Verification items for the finished model (mm, model axes). Face numbers are marked on the shaded views. A direction names the side the tool comes from. Round coordinates to 2 decimals unless told otherwise and drop trailing zeros. Loops run counter-clockwise (first coordinate to the right, second up) from the corner with the lowest first, then second, coordinate; pieces in that order, holes last. Notation, with made-up numbers: (19.5, -19.75) - (26.5, -19.75) arc R30 ccw to (26.5, 12.25) - close; hole circle Ø7 at (82, -11). An arc over 180 degrees is marked (long way). Use a Markdown table: item, result. Add a question column.
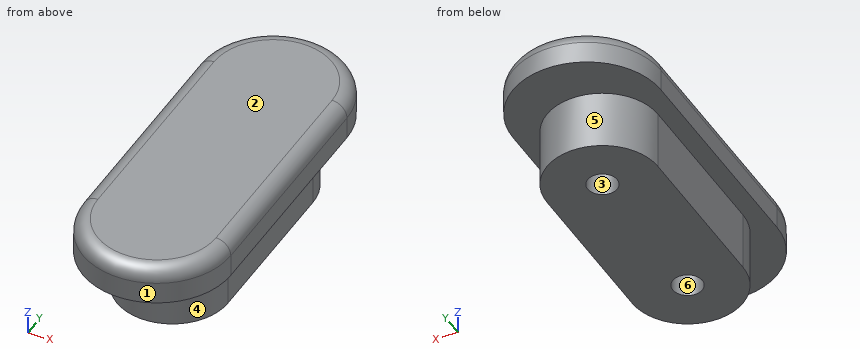
```python
from build123d import *

# Parameters (mm, degrees)
SKETCH_2_R      = 2
EXTRUDE_1_DEPTH = 8
EXTRUDE_2_DEPTH = 5
FILLET_1_R      = 2


with BuildPart() as part:
    # 草图2 → 凸台-拉伸1 (new body)
    with BuildSketch(Plane.XY):
        with BuildLine():
            Line((-7.5, -11), (-7.5, 11))
            ThreePointArc((-7.5, 11), (0, 18.5), (7.5, 11))
            Line((7.5, 11), (7.5, -11))
            ThreePointArc((7.5, -11), (0, -18.5), (-7.5, -11))
        make_face()
        with Locations((0, -11)):
            Circle(SKETCH_2_R, mode=Mode.SUBTRACT)
        with Locations((0, 11)):
            Circle(SKETCH_2_R, mode=Mode.SUBTRACT)
    extrude(amount=EXTRUDE_1_DEPTH)

    # 草图3 → 凸台-拉伸2 (add)
    with BuildSketch(Plane.XY.offset(8)):
        with BuildLine():
            Line((-10, -15), (-10, 15))
            ThreePointArc((-10, 15), (0, 25), (10, 15))
            Line((10, 15), (10, -15))
            ThreePointArc((10, -15), (0, -25), (-10, -15))
        make_face()
    extrude(amount=EXTRUDE_2_DEPTH)

    # 圆角1
    fillet_1_edges = [part.edges().sort_by_distance(p)[0] for p in [
        (0, -25, 13),
        (10, 0, 13),
        (0, 25, 13),
        (-10, 0, 13),
    ]]
    fillet(fillet_1_edges, radius=FILLET_1_R)


solid = part.part
```
Q1. Section check A-A on z = 7.5. Record the cut outline in (x, y), plus the area to 3 significant figures.
Q2. Thickness scan on line 1 along Y through (x, z) = (0, 3.5); line 2 along Y through (x, z) = (-1, 7.75); line 3 along Z through (x, y) = (-2.5, 19). Record the ranges inside material, lowest first.
Q3. Go/stop test with flat-tipped pins: pin 1 Ø4 at (x, z) = (4.5, 3.5) entering from +Y; pin 2 Ø1.5 at (y, z) = (2.5, 3) entering from -X; pin 3 Ø3 at (y, z) = (-17, 9.5) entering from -X. Record where each tip stops, or that it passes through.
Q4. Section check C-C on y = -4.5. Record the cut outline in (x, z).
Q5. Section check D-D on z = 11.5. Record the cut outline in (x, y), plus the area to 3 significant figures.
Q6. Release check for a two-part mould opening along Y. For the marked faces 1, 2 and 3 record: +Y half, -Y half, draft (parallel to the pull), parting line (faces both ways), or undercut.
Q7. Section check B-B on x = 0. Record the cut outline in (y, z), plus the area to 3 significant figures.
Q8. Set-up check for the marked faces 4, 5 and 6: record each of +Z, -Z, +X, -X, +Y, -Y from which the full face is reachable in a straight line by a thin tool's end or side.
Determined:
| question | item | result |
|---|---|---|
| 1 | outline | (-7.5, -11) arc R7.5 ccw to (7.5, -11) - (7.5, 11) arc R7.5 ccw to (-7.5, 11) - close; hole circle Ø4 at (0, -11); hole circle Ø4 at (0, 11) |
| 1 | area | 482 mm² |
| 2 | line 1 | y = -18.5 to -13, -9 to 9, 13 to 18.5 |
| 2 | line 2 | y = -18.43 to -12.73, -9.27 to 9.27, 12.73 to 18.43 |
| 2 | line 3 | z = 8 to 13 |
| 3 | pin 1 | stops at y = 18.07 |
| 3 | pin 2 | stops at x = -7.5 |
| 3 | pin 3 | stops at x = -9.99 |
| 4 | outline | (-10, 8) - (-7.5, 8) - (-7.5, 0) - (7.5, 0) - (7.5, 8) - (10, 8) - (10, 11) arc R2 ccw to (8, 13) - (-8, 13) arc R2 ccw to (-10, 11) - close |
| 5 | outline | (-9.94, -15) arc R9.94 ccw to (9.94, -15) - (9.94, 15) arc R9.94 ccw to (-9.94, 15) - close |
| 5 | area | 906 mm² |
| 6 | face 1 | -Y half |
| 6 | face 2 | draft |
| 6 | face 3 | undercut |
| 7 | outline | (-25, 8) - (-18.5, 8) - (-18.5, 0) - (-13, 0) - (-13, 8) - (-9, 8) - (-9, 0) - (9, 0) - (9, 8) - (13, 8) - (13, 0) - (18.5, 0) - (18.5, 8) - (25, 8) - (25, 11) arc R2 ccw to (23, 13) - (-23, 13) arc R2 ccw to (-25, 11) - close |
| 7 | area | 480 mm² |
| 8 | face 4 | -Z, -Y |
| 8 | face 5 | -Z, +Y |
| 8 | face 6 | -Z |
